from build123d import *

# Parameters (mm, degrees)
SKETCH1_W           = 42
SKETCH1_H           = 42
BOSS_EXTRUDE1_DEPTH = 32
CHAMFER1_SIZE       = 5
SKETCH2_R           = 11.05
BOSS_EXTRUDE2_DEPTH = 2
SKETCH3_R           = 2.5
BOSS_EXTRUDE3_DEPTH = 20
SKETCH4_R           = 1.6
CUT_EXTRUDE1_DEPTH  = 5


with BuildPart() as part:
    # Sketch1 → Boss-Extrude1 (new body)
    with BuildSketch(Plane(origin=(0, 0, 0), x_dir=(1, 0, 0), z_dir=(0, 1, 0))):
        Rectangle(SKETCH1_W, SKETCH1_H)
    extrude(amount=BOSS_EXTRUDE1_DEPTH)

    # Chamfer1
    chamfer1_edges = [part.edges().sort_by_distance(p)[0] for p in [
        (21, 16, 21),
        (-21, 16, 21),
        (-21, 16, -21),
        (21, 16, -21),
    ]]
    chamfer(chamfer1_edges, length=CHAMFER1_SIZE)

    # Sketch2 → Boss-Extrude2 (add)
    with BuildSketch(Plane(origin=(0, 32, 0), x_dir=(1, 0, 0), z_dir=(0, 1, 0))):
        Circle(SKETCH2_R)
    extrude(amount=BOSS_EXTRUDE2_DEPTH)

    # Sketch3 → Boss-Extrude3 (add)
    with BuildSketch(Plane(origin=(0, 34, 0), x_dir=(1, 0, 0), z_dir=(0, 1, 0))):
        Circle(SKETCH3_R)
    extrude(amount=BOSS_EXTRUDE3_DEPTH)

    # Sketch4 → Cut-Extrude1 (cut)
    with BuildSketch(Plane(origin=(0, 32, 0), x_dir=(1, 0, 0), z_dir=(0, 1, 0))):
        with Locations((-15.7, 15.7)):
            Circle(SKETCH4_R)
        with Locations((15.5, 15.7)):
            Circle(SKETCH4_R)
        with Locations((15.5, -15.5)):
            Circle(SKETCH4_R)
        with Locations((-15.7, -15.5)):
            Circle(SKETCH4_R)
    extrude(amount=-CUT_EXTRUDE1_DEPTH, mode=Mode.SUBTRACT)


solid = part.part
Verification items for the finished model (mm, model axes). A direction names the side the tool comes from. Coordinates: 2 decimals unless noted, no trailing zeros. Write each loop counter-clockwise with the first axis right and the second up, starting at its lowest first coordinate (ties: lowest second). Pieces come first, ordered by that corner, then holes. Notation, with made-up numbers: (-21, 72) -> (1, 72) arc R27 cw to (1, 96) -> close; hole circle Ø7 at (46, 25.25). An arc over 180 degrees is marked (long way). One line per item, written item: value. Start each with the question number.
Q1. Cross-section at B-B on z = 0. Enter the section's corners in (x, y).
Q2. Cross-section at A-A on x = 0. Enter the section's corners in (y, z), and give its area (3 significant figures).
Q3. Cross-section at D-D on x = -6. Enter the section's corners in (y, z), and give its area (3 significant figures).
Q4. Go/stop test with flat-tipped pins: P1, Ø2.5, axis at x = -15.7, z = -15.7, coming from the -Y side; P2, Ø1, axis at x = 15.5, z = 16, coming from the +Y side; P3, Ø1.5, axis at x = 3.5, y = 47.5, coming from the -Z side; P4, Ø1.6, axis at x = -15, z = 16, coming from the +Y side. Record where each tip stops, or that it passes through.
Q5. Cross-section at C-C on y = 18. Enter the section's corners in (x, z), and give its area (3 significant figures).
Q6. Thickness scan on L1, parallel to Z at x = 15.5, y = 29.4; L2, parallel to Z at x = 15, y = 28. Record the ranges inside material, lowest first. Write a range as from..to.
Q7. Access from +Z, -Z, +X, -X, +Y, -Y to the whole of each face (thin tool, end or side, straight path). Record for faces 1 (the flat face through (0, 54, 0)), 2 (the cylindrical face through (13.9, 29.54, -15.77)).
Q8. Mould release check, pull along Z, two halves, no side actions. Record for faces 3 (the cylindrical face through (-2.395, 32.986, 10.787)), 4 (the flat face through (0, 16, 21)), 5 (the flat face through (-16, 27, -16)): pulls with the +Z half, pulls with the -Z half, needs draft (parallel to the pull), parting line crosses it, or undercut.
Checked values:
1. outline: (-21, 0) -> (21, 0) -> (21, 32) -> (11.05, 32) -> (11.05, 34) -> (2.5, 34) -> (2.5, 54) -> (-2.5, 54) -> (-2.5, 34) -> (-11.05, 34) -> (-11.05, 32) -> (-21, 32) -> close
2. outline: (0, -21) -> (32, -21) -> (32, -11.05) -> (34, -11.05) -> (34, -2.5) -> (54, -2.5) -> (54, 2.5) -> (34, 2.5) -> (34, 11.05) -> (32, 11.05) -> (32, 21) -> (0, 21) -> close
2. area: 1,490 mm²
3. outline: (0, -21) -> (32, -21) -> (32, -9.28) -> (34, -9.28) -> (34, 9.28) -> (32, 9.28) -> (32, 21) -> (0, 21) -> close
3. area: 1,380 mm²
4. P1: stops at y = 0
4. P2: stops at y = 27
4. P3: passes through
4. P4: stops at y = 32
5. outline: (-21, -16) -> (-16, -21) -> (16, -21) -> (21, -16) -> (21, 16) -> (16, 21) -> (-16, 21) -> (-21, 16) -> close
5. area: 1,710 mm²
6. L1: z = -21..-17.3, -14.1..13.9, 17.1..21
6. L2: z = -21..-17.22, -14.18..13.98, 17.02..21
7. face 1: +Z, -Z, +X, -X, +Y
7. face 2: +Y
8. face 3: parting line crosses it
8. face 4: pulls with the +Z half
8. face 5: undercut
